Geometry check sheet. Reference: the model listing, model coordinates, mm. Give positions to 0.01 mm unless a question says otherwise; leave off trailing zeros. Write each loop counter-clockwise with the first axis right and the second up, starting at its lowest first coordinate (ties: lowest second). Pieces come first, ordered by that corner, then holes.
(1) Cross-section at C-C (z = 20). Record the boundary of the cut face in (x, y).
(2) Depth check by flat-ended pin: P1, Ø1.5, axis at y = 2.5, z = 6.5, coming from the +X side; P2, Ø5, axis at x = 1.5, z = 3.5, coming from the +Y side. Enter the tip coordinate at first touch or a pass-through.
(3) Mould release check, pull along X, two halves, no side actions. Record for faces 1 (the cylindrical face through (0.596, -2.685, 14.79)), 2 (the flat face through (1, -3, 0)), 3 (the conical face through (-0.61, 4.647, 22.395)): +X half, -X half, draft (parallel to the pull), parting line (faces both ways), or undercut.
(4) Cross-section at B-B (z = 6). Record the boundary of the cut face in (x, y).
(5) Thickness scan on line 1 along Y through (x, z) = (0, 17); line 2 along Y through (x, z) = (-0.75, 5); line 3 along X through (y, z) = (-2.5, 8.5). Record the ranges inside material, lowest first.
(6) Cross-section at A-A (x = 0). Record the boundary of the cut face in (y, z) (3 decimals), and give its area (3 significant figures).
```python
from build123d import *

# Parameters (mm, degrees)
F0_R     = 4.155
F1_DEPTH = 15
F1_TAPER = -4
F4_D     = 5.5


with BuildPart() as f1:
    # F0 (on Top) → F1 (new body)
    with BuildSketch(Plane.XY):
        Circle(F0_R)
    extrude(amount=F1_DEPTH, taper=F1_TAPER)

    # F2: F1 across face


with BuildPart() as f1_1:
    add(f1.part)
    add(f1.part.mirror(Plane.XY.offset(15)))

    # F4 (through all)
    with Locations(Plane.XY.offset(30)):
        with Locations((0, 0)):
            Hole(F4_D / 2)


solid = f1_1.part
```
Reply:
1. outline: circle Ø9.71 at (0, 0); hole circle Ø5.5 at (0, 0)
2. P1: stops at x = 4.27
2. P2: stops at y = 4.54
3. face 1: undercut
3. face 2: draft
3. face 3: parting line
4. outline: circle Ø9.15 at (0, 0); hole circle Ø5.5 at (0, 0)
5. line 1: y = -5.06 to -2.75, 2.75 to 5.06
5. line 2: y = -4.44 to -2.65, 2.65 to 4.44
5. line 3: x = -4.04 to -1.15, 1.15 to 4.04
6. outline: (-5.204, 15) - (-4.155, 0) - (-2.75, 0) - (-2.75, 30) - (-4.155, 30) - close; (2.75, 0) - (4.155, 0) - (5.204, 15) - (4.155, 30) - (2.75, 30) - close
6. area: 116 mm2
